Verification items for the finished model (mm, model axes). A direction names the side the tool comes from. Coordinates: 2 decimals unless noted, no trailing zeros. Order: outer loops, then holes, each group sorted by start corner. A loop starts at its lowest first (then second) coordinate and runs counter-clockwise, first axis right, second up. Notation, with made-up numbers: M -23.75,27 L -1.75,27 A23 cw -1.75,59 Z; hole C 2,80 d10. An arc over 180 degrees is marked long. Use one line per item in the form item = value. Start each with the question number.
```python
from build123d import *

# Parameters (mm, degrees)
SKETCH1_W           = 90
SKETCH1_H           = 70
BOSS_EXTRUDE1_DEPTH = 12.5
SKETCH3_W           = 90
SKETCH3_H           = 15
BOSS_EXTRUDE2_DEPTH = 15
SKETCH4_R           = 1.25
SKETCH4_W           = 22
SKETCH4_H           = 42
CUT_EXTRUDE1_DEPTH  = 64.294944506
SKETCH7_W           = 90
SKETCH7_H           = 70
SKETCH7_W_2         = 20
SKETCH7_H_2         = 20
BOSS_EXTRUDE3_DEPTH = 5
SKETCH8_R           = 26.514354508
SKETCH8_R_2         = 2.5
BOSS_EXTRUDE4_DEPTH = 5
SKETCH12_W          = 22
SKETCH12_H          = 14
CUT_EXTRUDE3_DEPTH  = 69.23672032
SKETCH16_W          = 26
SKETCH16_H          = 70
CUT_EXTRUDE5_DEPTH  = 69.23672032
BOSS_EXTRUDE5_START = 15
SKETCH17_R          = 1.25
BOSS_EXTRUDE5_DEPTH = 15
SKETCH18_R          = 1.5
CUT_EXTRUDE6_DEPTH  = 30


with BuildPart() as part:
    # Sketch1 → Boss-Extrude1 (new body)
    with BuildSketch(Plane(origin=(0, 0, 0), x_dir=(1, 0, 0), z_dir=(0, 1, 0))):
        Rectangle(SKETCH1_W, SKETCH1_H)
    extrude(amount=BOSS_EXTRUDE1_DEPTH)

    # Sketch3 → Boss-Extrude2 (add)
    with BuildSketch(Plane.XZ):
        Rectangle(SKETCH3_W, SKETCH3_H)
    extrude(amount=BOSS_EXTRUDE2_DEPTH)

    # Sketch4 → Cut-Extrude1 (cut, through all)
    with BuildSketch(Plane(origin=(0, 12.5, 0), x_dir=(1, 0, 0), z_dir=(0, 1, 0))):
        with Locations(Location((-5, 24, 0), (0, 0, 270))):
            Circle(SKETCH4_R)
        with Locations(Location((5, 24, 0), (0, 0, 270))):
            Circle(SKETCH4_R)
        with Locations(Location((5, -24, 0), (0, 0, 270))):
            Circle(SKETCH4_R)
        with Locations(Location((-5, -24, 0), (0, 0, 270))):
            Circle(SKETCH4_R)
        Rectangle(SKETCH4_W, SKETCH4_H)
    extrude(amount=-CUT_EXTRUDE1_DEPTH, mode=Mode.SUBTRACT)

    # Sketch7 → Boss-Extrude3 (add)
    with BuildSketch(Plane.XZ.offset(15)):
        Rectangle(SKETCH7_W, SKETCH7_H)
        Rectangle(SKETCH7_W_2, SKETCH7_H_2, mode=Mode.SUBTRACT)
    extrude(amount=BOSS_EXTRUDE3_DEPTH)

    # Sketch8 → Boss-Extrude4 (add)
    with BuildSketch(Plane.XZ.offset(20)):
        with Locations(Location((0, 0, 0), (0, 0, 270))):
            Circle(SKETCH8_R)
        with Locations(Location((0, 0, 0), (0, 0, 270))):
            Circle(SKETCH8_R_2, mode=Mode.SUBTRACT)
    extrude(amount=BOSS_EXTRUDE4_DEPTH)

    # Sketch12 → Cut-Extrude3 (cut, through all)
    with BuildSketch(Plane(origin=(0, 12.5, 0), x_dir=(1, 0, 0), z_dir=(0, 1, 0))):
        with Locations((0, -28)):
            Rectangle(SKETCH12_W, SKETCH12_H)
    extrude(amount=-CUT_EXTRUDE3_DEPTH, mode=Mode.SUBTRACT)

    # Sketch16 → Cut-Extrude5 (cut, through all)
    with BuildSketch(Plane(origin=(0, 12.5, 0), x_dir=(1, 0, 0), z_dir=(0, 1, 0))):
        with Locations((-32, 0)):
            Rectangle(SKETCH16_W, SKETCH16_H)
        with Locations((32, 0)):
            Rectangle(SKETCH16_W, SKETCH16_H)
    extrude(amount=-CUT_EXTRUDE5_DEPTH, mode=Mode.SUBTRACT)

    # Sketch17 → Boss-Extrude5 (add)
    with BuildSketch(Plane(origin=(0, 12.5, 0), x_dir=(1, 0, 0), z_dir=(0, 1, 0)).offset(BOSS_EXTRUDE5_START)):
        Polygon((19, 35), (-19, 35), (-19, -35), (-11, -35), (-11, 21), (11, 21), (11, -35), (19, -35), align=None)
        with Locations(Location((5, 24, 0), (0, 0, 270))):
            Circle(SKETCH17_R, mode=Mode.SUBTRACT)
        with Locations(Location((-5, 24, 0), (0, 0, 270))):
            Circle(SKETCH17_R, mode=Mode.SUBTRACT)
    extrude(amount=-BOSS_EXTRUDE5_DEPTH)

    # Sketch18 → Cut-Extrude6 (cut)
    with BuildSketch(Plane(origin=(0, 27.5, 0), x_dir=(1, 0, 0), z_dir=(0, 1, 0))):
        with Locations(Location((-5, 24, 0), (0, 0, 270))):
            Circle(SKETCH18_R)
        with Locations(Location((5, 24, 0), (0, 0, 270))):
            Circle(SKETCH18_R)
    extrude(amount=-CUT_EXTRUDE6_DEPTH, mode=Mode.SUBTRACT)


solid = part.part
```
1. Cross-section at D-D on z = 1.5. Enter the section's corners in (x, y), and give its area (3 significant figures).
2. Release check for a two-part mould opening along X. For faces 5 (the flat face through (-19, 7, 0)), 6 (the flat face through (11, -19, 27)), 7 (the flat face through (0, -20, -28)), 8 (the flat face through (0, 14, -21)) record: pulls with the +X half, pulls with the -X half, needs draft (parallel to the pull), parting line crosses it, or undercut.
3. Tool access check on faces 1 (the flat face through (15, -20, 29)), 2 (the flat face through (-15, 0, 21)), 3 (the flat face through (-11, 11, 7)), 4 (the flat face through (10, -17, 0)). Record the directions out of +Z, -Z, +X, -X, +Y, -Y that give a thin tool (end or side, any length) a straight path to the whole face; none if there is none.
4. Depth check by flat-ended pin: P1, Ø12, axis at x = 8, z = 22, coming from the +Y side; P2, Ø1.5, axis at x = 4.5, y = -18.5, coming from the +Z side; P3, Ø16, axis at x = 0.5, z = -3, coming from the +Y side; P4, Ø6.5, axis at x = 16.5, z = 27, coming from the -Y side. Enter the tip coordinate at first touch or a pass-through.
5. Cross-section at C-C on y = 8. Enter the section's corners in (x, z), and give its area (3 significant figures).
6. Cross-section at A-A on z = 26. Enter the section's corners in (x, y).
7. Cross-section at B-B on x = 0. Enter the section's corners in (y, z).
8. Material ranges on line 1 along X through (y, z) = (13.25, -24); line 2 along Y through (x, z) = (13, 12); line 3 along Y through (x, z) = (17.5, -26), recorded low to high.
Final values:
q1.outline = M -19,-25 L -2,-25 L -2,-20 L -10,-20 L -10,-15 L -11,-15 L -11,27.5 L -19,27.5 Z; M 2,-25 L 19,-25 L 19,27.5 L 11,27.5 L 11,-15 L 10,-15 L 10,-20 L 2,-20 Z
q1.area = 940 mm2
q2.face_5 = pulls with the -X half
q2.face_6 = undercut
q2.face_7 = needs draft
q2.face_8 = undercut
q3.face_1 = +Z, +X, -Y
q3.face_2 = +Z, +X, -X
q3.face_3 = +Z, +Y
q3.face_4 = +Y
q4.P1 = 27.5
q4.P2 = 21
q4.P3 = -15
q4.P4 = -20
q5.outline = M -19,-35 L 19,-35 L 19,35 L 11,35 L 11,-21 L -11,-21 L -11,35 L -19,35 Z; hole C -5,-24 d3; hole C 5,-24 d3
q5.area = 1,410 mm2
q6.outline = M -19,-20 L -11,-20 L -11,-15 L -19,-15 Z; M -19,0 L -11,0 L -11,27.5 L -19,27.5 Z; M 11,-20 L 19,-20 L 19,-15 L 11,-15 Z; M 11,0 L 19,0 L 19,27.5 L 11,27.5 Z
q7.outline = M -25,-26.51 L -20,-26.51 L -20,-35 L -15,-35 L -15,-10 L -20,-10 L -20,-2.5 L -25,-2.5 Z; M -25,2.5 L -20,2.5 L -20,10 L -15,10 L -15,21 L -25,21 Z; M 0,-35 L 27.5,-35 L 27.5,-21 L 0,-21 Z
q8.line_1 = -19 to -6.5, -3.5 to 3.5, 6.5 to 19
q8.line_2 = -25 to -15, 0 to 27.5
q8.line_3 = -20 to -15, 0 to 27.5
